Geometry: see drawing. Coordinates: mm, zero at the bounding-box minimum. A direction names the side the tool comes from. Give positions to 0.01 mm unless a question says otherwise; leave off trailing zeros. Write each loop counter-clockwise with the first axis right and the second up, starting at its lowest first coordinate (ties: lowest second). Pieces come first, ordered by that corner, then holes. Notation, with made-up numbers: (70.25, 12) -> (98.25, 12) arc R10 ccw to (98.25, 29) -> close; hole circle Ø7 at (50, 85). An arc over 180 degrees is marked (long way). Use one line per item in the form item = value. Start each with the question number.
(1) First-contact query: P1, Ø1, axis at y = 11.5, z = 5, coming from the +X side; P2, Ø1.5, axis at y = 15, z = 2.5, coming from the -X side; P3, Ø2.5, axis at x = 5, y = 4.5, coming from the -Z side; P4, Ø3.5, axis at y = 8.5, z = 8.5, coming from the -X side. Flat tips, straight axial feed; report the tip coordinate or a pass-through.
(2) Cut plane B-B, the plane x = 50. Output: boundary loops of the cut face in (y, z).
(3) Material intervals for line 1 along Y through (x, z) = (50, 2.4); line 2 along Y through (x, z) = (5, 2.8); line 3 along Z through (x, y) = (9, 15), sorted ascending. Write a range as from..to.
(4) Cut plane D-D, the plane y = 22.5. Output: boundary loops of the cut face in (x, z), and give its area (3 significant figures).
(5) Cut plane C-C, the plane x = 5. Output: boundary loops of the cut face in (y, z).
(6) Cut plane A-A, the plane y = 4.5. Output: boundary loops of the cut face in (x, z).
(7) Set-up query: the marked faces 1, 2, 3, 4 and 5. Return all of +Z, -Z, +X, -X, +Y, -Y with unobstructed straight access to the full face (end or side cutting, diameter ignored); none if empty.
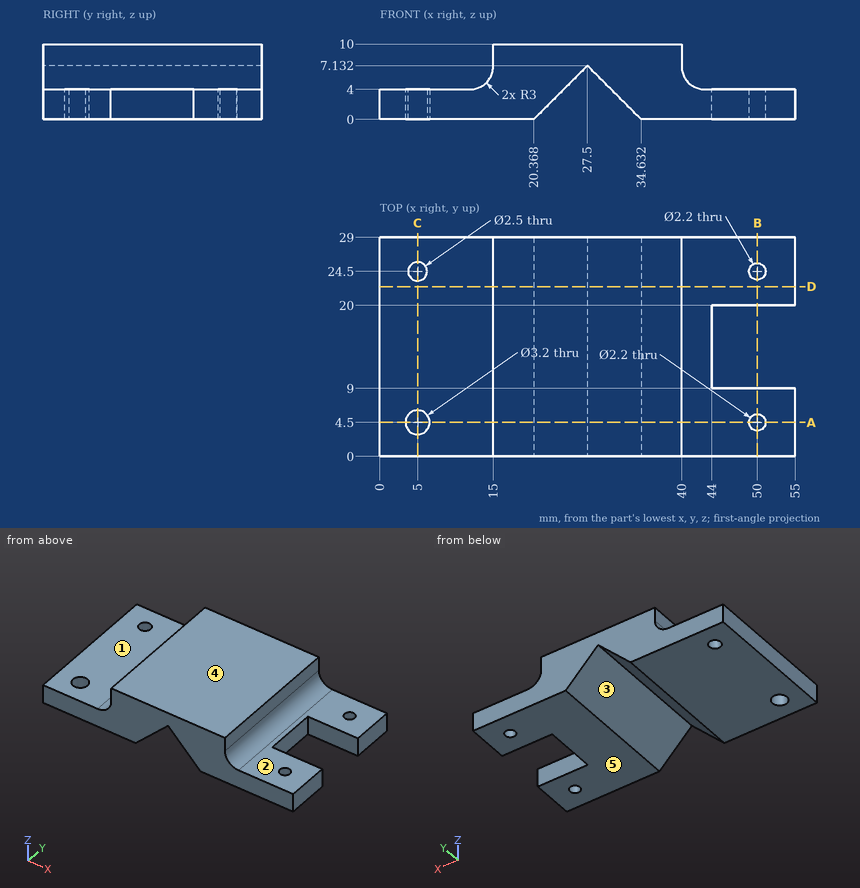
Geometry says:
q1.P1 = 41.34
q1.P2 = 0
q1.P3 = through
q1.P4 = 14.99
q2.outline = (0, 0) -> (3.4, 0) -> (3.4, 4) -> (0, 4) -> close; (5.6, 0) -> (9, 0) -> (9, 4) -> (5.6, 4) -> close; (20, 0) -> (23.4, 0) -> (23.4, 4) -> (20, 4) -> close; (25.6, 0) -> (29, 0) -> (29, 4) -> (25.6, 4) -> close
q3.line_1 = 0..3.4, 5.6..9, 20..23.4, 25.6..29
q3.line_2 = 0..2.9, 6.1..23.25, 25.75..29
q3.line_3 = 0..4
q4.outline = (0, 0) -> (20.37, 0) -> (27.5, 7.13) -> (34.63, 0) -> (55, 0) -> (55, 4) -> (43, 4) arc R3 cw to (40, 7) -> (40, 10) -> (15, 10) -> (15, 7) arc R3 cw to (12, 4) -> (0, 4) -> close
q4.area = 323 mm^2
q5.outline = (0, 0) -> (2.9, 0) -> (2.9, 4) -> (0, 4) -> close; (6.1, 0) -> (23.25, 0) -> (23.25, 4) -> (6.1, 4) -> close; (25.75, 0) -> (29, 0) -> (29, 4) -> (25.75, 4) -> close
q6.outline = (0, 0) -> (3.4, 0) -> (3.4, 4) -> (0, 4) -> close; (6.6, 0) -> (20.37, 0) -> (27.5, 7.13) -> (34.63, 0) -> (48.9, 0) -> (48.9, 4) -> (43, 4) arc R3 cw to (40, 7) -> (40, 10) -> (15, 10) -> (15, 7) arc R3 cw to (12, 4) -> (6.6, 4) -> close; (51.1, 0) -> (55, 0) -> (55, 4) -> (51.1, 4) -> close
q7.face_1 = +Z, -X, +Y, -Y
q7.face_2 = +Z, +X, +Y, -Y
q7.face_3 = -Z, +Y, -Y
q7.face_4 = +Z, +X, -X, +Y, -Y
q7.face_5 = -Z, +X, -X, +Y, -Y
